The listing builds one solid part. Answer for the finished solid, in the listing's coordinates (mm). A direction names the side the tool comes from. Give positions to 0.01 mm unless a question says otherwise; leave off trailing zeros. Loops run counter-clockwise (first coordinate to the right, second up) from the corner with the lowest first, then second, coordinate; pieces in that order, holes last.
Item 1: Each of these flat-tipped pins is pushed along its axis until it touches: pin 1 Ø3 at (x, z) = (7, -2.5) entering from +Y; pin 2 Ø7 at (x, z) = (-0.5, -2) entering from -Y; pin 3 Ø6 at (y, z) = (13, -3.5) entering from +X; pin 4 Ø10 at (y, z) = (5.5, 0) entering from -X. Where does it stop, or does it pass through?
Item 2: Consider line 1 along X through (y, z) = (12.5, 0); line 2 along Z through (x, y) = (0, 0.9); line 3 along Y through (x, z) = (-8, -3). Determine where each line is inside the solid, lowest interval first.
Item 3: Section B-B, the plane y = 8 is taken. Give the vertices of the cut face in (x, z).
Item 4: Section A-A, the plane x = 0 is taken. Give the vertices of the cut face in (y, z), and give its area (3 significant figures).
Item 5: The mould has two halves that part along Z. Classify faces 1 (the face through (1, 2.2, 5)), 2 (the face through (-7.328, 2.218, -4.308)), 3 (the face through (6, 0, -4)): pulls with the +Z half, pulls with the -Z half, needs draft (parallel to the pull), parting line crosses it, or undercut.
Item 6: A tool of negligible diameter and unlimited length cuts with its end or side. For faces 4 (the face through (-1.46, 1.08, -6.59)), 5 (the face through (6.4, 4.5, -0.1)), 6 (the face through (0, 2, 8.5)), from which of +Z, -Z, +X, -X, +Y, -Y can it reach the whole face along a straight path? Write none if from no direction.
from build123d import *

# Parameters (mm, degrees)
SKETCH_1_R          = 4.65
EXTRUDE_1_DEPTH     = 17
SKETCH_2_R          = 6
CUT_EXTRUDE_1_DEPTH = 12.5
SKETCH_3_R          = 6.75
SKETCH_3_R_2        = 4.65
CUT_EXTRUDE_2_DEPTH = 2.2
CHAMFER_1_SIZE      = 0.5
CUT_EXTRUDE_3_DEPTH = 18


with BuildPart() as part:
    # Эскиз1 → Бобышка-Вытянуть1 (new body)
    with BuildSketch(Plane(origin=(0, 0, 0), x_dir=(1, 0, 0), z_dir=(0, 1, 0))):
        Polygon((9.814954576, 0), (4.907477288, 8.5), (-4.907477288, 8.5), (-9.814954576, 0), (-4.907477288, -8.5), (4.907477288, -8.5), align=None)
        Circle(SKETCH_1_R, mode=Mode.SUBTRACT)
    extrude(amount=EXTRUDE_1_DEPTH)

    # Эскиз2 → Вырез-Вытянуть1 (cut)
    with BuildSketch(Plane(origin=(0, 17, 0), x_dir=(1, 0, 0), z_dir=(0, 1, 0))):
        Polygon((-4.907477288, -8.5), (4.907477288, -8.5), (9.814954576, 0), (4.907477288, 8.5), (-4.907477288, 8.5), (-9.814954576, 0), align=None)
        Circle(SKETCH_2_R, mode=Mode.SUBTRACT)
    extrude(amount=-CUT_EXTRUDE_1_DEPTH, mode=Mode.SUBTRACT)

    # Эскиз3 → Вырез-Вытянуть2 (cut)
    with BuildSketch(Plane.XZ):
        Circle(SKETCH_3_R)
        Circle(SKETCH_3_R_2, mode=Mode.SUBTRACT)
    extrude(amount=-CUT_EXTRUDE_2_DEPTH, mode=Mode.SUBTRACT)

    # Фаска1
    chamfer_1_edges = [part.edges().sort_by_distance(p)[0] for p in [
        (-6, 17, 0),
    ]]
    chamfer(chamfer_1_edges, length=CHAMFER_1_SIZE)

    # Эскиз4 → Вырез-Вытянуть3 (cut, through all)
    with BuildSketch(Plane.XZ):
        with BuildLine():
            ThreePointArc((-9.749337579, -0.113651973), (-9.75, 0), (-9.749337579, 0.113651973))
            Line((-9.749337579, 0.113651973), (-9.814954576, 0))
            Line((-9.814954576, 0), (-9.749337579, -0.113651973))
        make_face()
        with BuildLine():
            ThreePointArc((-4.973094285, 8.386348027), (-4.875, 8.443747687), (-4.776243294, 8.5))
            Line((-4.776243294, 8.5), (-4.907477288, 8.5))
            Line((-4.907477288, 8.5), (-4.973094285, 8.386348027))
        make_face()
        with BuildLine():
            ThreePointArc((4.776243294, 8.5), (4.875, 8.443747687), (4.973094285, 8.386348027))
            Line((4.973094285, 8.386348027), (4.907477288, 8.5))
            Line((4.907477288, 8.5), (4.776243294, 8.5))
        make_face()
        with BuildLine():
            ThreePointArc((9.749337579, 0.113651973), (9.749834393, 0.056826952), (9.75, 0))
            ThreePointArc((9.75, 0), (9.749834393, -0.056826952), (9.749337579, -0.113651973))
            Line((9.749337579, -0.113651973), (9.814954576, 0))
            Line((9.814954576, 0), (9.749337579, 0.113651973))
        make_face()
        with BuildLine():
            Line((4.907477288, -8.5), (4.973094285, -8.386348027))
            ThreePointArc((4.973094285, -8.386348027), (4.875, -8.443747687), (4.776243294, -8.5))
            Line((4.776243294, -8.5), (4.907477288, -8.5))
        make_face()
        with BuildLine():
            Line((-4.907477288, -8.5), (-4.776243294, -8.5))
            ThreePointArc((-4.776243294, -8.5), (-4.875, -8.443747687), (-4.973094285, -8.386348027))
            Line((-4.973094285, -8.386348027), (-4.907477288, -8.5))
        make_face()
    extrude(amount=-CUT_EXTRUDE_3_DEPTH, mode=Mode.SUBTRACT)


solid = part.part
Worked answers:
1. pin 1: stops at y = 16.57
1. pin 2: stops at y = 2.2
1. pin 3: stops at x = 5.98
1. pin 4: stops at x = -9.75
2. line 1: x = -6 to -4.65, 4.65 to 6
2. line 2: z = -8.5 to -6.75, 6.75 to 8.5
2. line 3: y = 0 to 4.5
3. outline: circle Ø12 at (0, 0); hole circle Ø9.3 at (0, 0)
4. outline: (0, -8.5) - (4.5, -8.5) - (4.5, -6) - (16.5, -6) - (17, -5.5) - (17, -4.65) - (2.2, -4.65) - (2.2, -6.75) - (0, -6.75) - close; (0, 6.75) - (2.2, 6.75) - (2.2, 4.65) - (17, 4.65) - (17, 5.5) - (16.5, 6) - (4.5, 6) - (4.5, 8.5) - (0, 8.5) - close
4. area: 58.9 mm2
5. face 1: undercut
5. face 2: pulls with the -Z half
5. face 3: needs draft
6. face 4: -Y
6. face 5: +Y
6. face 6: +Z, +X, -X, +Y, -Y
